Read the model definition and answer for the solid it produces. Units are mm, in the model's axes. A direction names the side the tool comes from. Give positions to 0.01 mm unless a question says otherwise; leave off trailing zeros. Loops run counter-clockwise (first coordinate to the right, second up) from the corner with the lowest first, then second, coordinate; pieces in that order, holes last. Notation, with made-up numbers: (45, 56) - (71, 56) arc R18 ccw to (71, 69) - close; hole circle Ø4 at (56.5, 33). An arc over 180 degrees is marked (long way). Write item = value, one per line.
```python
from build123d import *

# Parameters (mm, degrees)
RESSALTO_EXTRUS_O1_DEPTH   = 27.5
ESBO_O6_R                  = 1.65
CORTE_EXTRUS_O3_DEPTH      = 6
CORTE_EXTRUS_O3_DEPTH_BACK = 10
CORTE_EXTRUS_O4_DEPTH      = 3
CORTE_EXTRUS_O4_DEPTH_BACK = 3
CORTE_EXTRUS_O5_DEPTH      = 3
ESBO_O10_W                 = 1.5
ESBO_O10_H                 = 5
RESSALTO_EXTRUS_O3_DEPTH   = 7


with BuildPart() as part:
    # Esbo_o1 → Ressalto-extrus_o1 (new body, symmetric)
    with BuildSketch(Plane.XY):
        with BuildLine():
            Line((0, 35), (0, -35))
            Line((0, -35), (13.5, -35))
            ThreePointArc((13.5, -35), (15.581665999, -34.780933834), (17.572127481, -34.133333333))
            Line((17.572127481, -34.133333333), (16.554095611, -31.85))
            ThreePointArc((16.554095611, -31.85), (6, -25), (16.554095611, -18.15))
            Line((16.554095611, -18.15), (17.572127481, -15.866666667))
            ThreePointArc((17.572127481, -15.866666667), (15.581665999, -15.219066166), (13.5, -15))
            Line((13.5, -15), (6, -15))
            Line((6, -15), (6, 15))
            Line((6, 15), (13.5, 15))
            ThreePointArc((13.5, 15), (15.581665999, 15.219066166), (17.572127481, 15.866666667))
            Line((17.572127481, 15.866666667), (16.554095611, 18.15))
            ThreePointArc((16.554095611, 18.15), (6, 25), (16.554095611, 31.85))
            Line((16.554095611, 31.85), (17.572127481, 34.133333333))
            ThreePointArc((17.572127481, 34.133333333), (15.581665999, 34.780933834), (13.5, 35))
            Line((13.5, 35), (0, 35))
        make_face()
    extrude(amount=RESSALTO_EXTRUS_O1_DEPTH, both=True)

    # Esbo_o6 → Corte-extrus_o3 (cut, two sides)
    with BuildSketch(Plane(origin=(6, 0, 0), x_dir=(0, 0, -1), z_dir=(1, 0, 0))) as corte_extrus_o3_sk:
        with Locations((-20, 15)):
            Circle(ESBO_O6_R)
        with Locations((20, -15)):
            Circle(ESBO_O6_R)
        with Locations((10, -15)):
            Circle(ESBO_O6_R)
        with Locations((-10, 15)):
            Circle(ESBO_O6_R)
        with Locations((10, 15)):
            Circle(ESBO_O6_R)
        with Locations((20, 15)):
            Circle(ESBO_O6_R)
        with Locations((-10, -15)):
            Circle(ESBO_O6_R)
        with Locations((-20, -15)):
            Circle(ESBO_O6_R)
        with Locations((0, 11)):
            Circle(ESBO_O6_R)
        Circle(ESBO_O6_R)
        with Locations((0, -11)):
            Circle(ESBO_O6_R)
    extrude(amount=CORTE_EXTRUS_O3_DEPTH, mode=Mode.SUBTRACT)
    extrude(corte_extrus_o3_sk.sketch, amount=-CORTE_EXTRUS_O3_DEPTH_BACK, mode=Mode.SUBTRACT)

    # Esbo_o8 → Corte-extrus_o4 (cut, two sides)
    with BuildSketch(Plane(origin=(6, 0, 0), x_dir=(0, 0, -1), z_dir=(1, 0, 0))) as corte_extrus_o4_sk:
        Polygon((-20, 11.824573519), (-17.25, 13.41228676), (-17.25, 16.58771324), (-20, 18.175426481), (-22.75, 16.58771324), (-22.75, 13.41228676), align=None)
        Polygon((-10, 11.824573519), (-7.25, 13.41228676), (-7.25, 16.58771324), (-10, 18.175426481), (-12.75, 16.58771324), (-12.75, 13.41228676), align=None)
        Polygon((-12.75, -13.41228676), (-10, -11.824573519), (-7.25, -13.41228676), (-7.25, -16.58771324), (-10, -18.175426481), (-12.75, -16.58771324), align=None)
        Polygon((-22.75, -13.41228676), (-20, -11.824573519), (-17.25, -13.41228676), (-17.25, -16.58771324), (-20, -18.175426481), (-22.75, -16.58771324), align=None)
        Polygon((20, -11.824573519), (17.25, -13.41228676), (17.25, -16.58771324), (20, -18.175426481), (22.75, -16.58771324), (22.75, -13.41228676), align=None)
        Polygon((10, -11.824573519), (7.25, -13.41228676), (7.25, -16.58771324), (10, -18.175426481), (12.75, -16.58771324), (12.75, -13.41228676), align=None)
        Polygon((12.75, 13.41228676), (10, 11.824573519), (7.25, 13.41228676), (7.25, 16.58771324), (10, 18.175426481), (12.75, 16.58771324), align=None)
        Polygon((22.75, 13.41228676), (20, 11.824573519), (17.25, 13.41228676), (17.25, 16.58771324), (20, 18.175426481), (22.75, 16.58771324), align=None)
    extrude(amount=CORTE_EXTRUS_O4_DEPTH, mode=Mode.SUBTRACT)
    extrude(corte_extrus_o4_sk.sketch, amount=-CORTE_EXTRUS_O4_DEPTH_BACK, mode=Mode.SUBTRACT)

    # Esbo_o9 → Corte-extrus_o5 (cut)
    with BuildSketch(Plane.ZY):
        Polygon((3.175426481, 11), (1.58771324, 13.75), (-1.58771324, 13.75), (-3.175426481, 11), (-1.58771324, 8.25), (1.58771324, 8.25), align=None)
        Polygon((3.175426481, 0), (1.58771324, 2.75), (-1.58771324, 2.75), (-3.175426481, 0), (-1.58771324, -2.75), (1.58771324, -2.75), align=None)
        Polygon((3.175426481, -11), (1.58771324, -8.25), (-1.58771324, -8.25), (-3.175426481, -11), (-1.58771324, -13.75), (1.58771324, -13.75), align=None)
    extrude(amount=-CORTE_EXTRUS_O5_DEPTH, mode=Mode.SUBTRACT)

    # Esbo_o10 → Ressalto-extrus_o3 (add)
    with BuildSketch(Plane.ZY):
        with Locations((-26.75, 25)):
            Rectangle(ESBO_O10_W, ESBO_O10_H)
        with Locations((26.75, 25)):
            Rectangle(ESBO_O10_W, ESBO_O10_H)
        with Locations((26.75, -25)):
            Rectangle(ESBO_O10_W, ESBO_O10_H)
        with Locations((-26.75, -25)):
            Rectangle(ESBO_O10_W, ESBO_O10_H)
    extrude(amount=-RESSALTO_EXTRUS_O3_DEPTH)


solid = part.part
```
1) A cutting plane is placed at B-B on y = -25. Determine the outline of the cut face in (x, z).
Output:
outline = (0, -27.5) - (7, -27.5) - (7, -26) - (6, -26) - (6, 26) - (7, 26) - (7, 27.5) - (0, 27.5) - close
2) Each of these flat-tipped pins is pushed along its axis until it touches: P1, Ø4.5, axis at y = 0, z = 0, coming from the +X side; P2, Ø6, axis at y = -15, z = 9.5, coming from the +X side; P3, Ø1.6, axis at y = 25.5, z = -27, coming from the +X side. Where does it stop, or does it pass through?
Output:
P1 = 6
P2 = 17.57
P3 = 7
3) A tool of negligible diameter and unlimited length cuts with its end or side. For faces 1 (the face through (17.06, 32.98, 0.39)), 2 (the face through (3, -16.4, 21.2)), 3 (the face through (4.52, 12.61, 18.64)), 4 (the face through (1.479, 1.394, -2.37)), from which of +Z, -Z, +X, -X, +Y, -Y can it reach the whole face along a straight path? Write none if from no direction.
Output:
face_1 = +Z, -Z, +X
face_2 = none
face_3 = +X
face_4 = -X
4) A cutting plane is placed at A-A on z = -4.5. Determine the outline of the cut face in (x, y).
Output:
outline = (0, -35) - (13.5, -35) arc R10 ccw to (17.57, -34.13) - (16.55, -31.85) arc R7.5 cw (long way) to (16.55, -18.15) - (17.57, -15.87) arc R10 ccw to (13.5, -15) - (6, -15) - (6, 15) - (13.5, 15) arc R10 ccw to (17.57, 15.87) - (16.55, 18.15) arc R7.5 cw (long way) to (16.55, 31.85) - (17.57, 34.13) arc R10 ccw to (13.5, 35) - (0, 35) - close
5) Find the intervals of material crossed by probe 1 along Y at (x, z) = (13.25, -21); probe 2 along Y at (x, z) = (4.6, 0); probe 3 along Y at (x, z) = (2.3, -20), in increasing order.
Output:
probe_1 = -35 to -32.5, -17.5 to -15, 15 to 17.5, 32.5 to 35
probe_2 = -35 to -12.65, -9.35 to -1.65, 1.65 to 9.35, 12.65 to 35
probe_3 = -35 to -16.65, -13.35 to 13.35, 16.65 to 35
